from build123d import *

# Parameters (mm, degrees)
BOSS_EXTRUDE1_DEPTH     = 70.5
CUT_EXTRUDE1_DEPTH      = 142.707445111
CUT_EXTRUDE1_DEPTH_BACK = 142.707445111
SKETCH2_R               = 2.5
FILLET1_R               = 1


with BuildPart() as part:
    # Sketch1 → Boss-Extrude1 (new, symmetric)
    with BuildSketch(Plane.XY):
        Polygon((-10, 10), (-3, 10), (-3, 8.272610059), (-5.783778863, 8.272610059), (-5.783778863, 6.747994248), (-3, 4.550753814), (3, 4.550753814), (5.783778863, 6.747994248), (5.783778863, 8.272610059), (3, 8.272610059), (3, 10), (10, 10), (10, 3), (8.272610059, 3), (8.272610059, 5.783778863), (6.747994248, 5.783778863), (4.55, 3.000595152), (4.55, -2.999404848), (6.747994248, -5.783778863), (8.272610059, -5.783778863), (8.272610059, -3), (10, -3), (10, -10), (3, -10), (3, -8.272610059), (5.783778863, -8.272610059), (5.783778863, -6.747994248), (2.999404848, -4.55), (-3.000595152, -4.55), (-5.783778863, -6.747994248), (-5.783778863, -8.272610059), (-3, -8.272610059), (-3, -10), (-10, -10), (-10, -3), (-8.272610059, -3), (-8.272610059, -5.783778863), (-6.747994248, -5.783778863), (-4.55, -3.000595152), (-4.55, 2.999404848), (-6.747994248, 5.783778863), (-8.272610059, 5.783778863), (-8.272610059, 3), (-10, 3), align=None)
    extrude(amount=BOSS_EXTRUDE1_DEPTH, both=True)

    # Sketch2 → Cut-Extrude1 (cut, two sides: drawn at the far end of the back side and taken through both)
    with BuildSketch(Plane.XY.offset(70.5).offset(-CUT_EXTRUDE1_DEPTH_BACK)):
        Circle(SKETCH2_R)
    extrude(amount=CUT_EXTRUDE1_DEPTH + CUT_EXTRUDE1_DEPTH_BACK, mode=Mode.SUBTRACT)

    # Fillet1
    fillet1_edges = [part.edges().sort_by_distance(p)[0] for p in [
        (-10, 10, 0),
        (10, 10, 0),
        (10, -10, 0),
        (-10, -10, 0),
    ]]
    fillet(fillet1_edges, radius=FILLET1_R)


solid = part.part
CAD build for the part. Positions are in the model's coordinates, mm. A direction names the side the tool comes from. Round coordinates to 2 decimals unless told otherwise and drop trailing zeros. Loops run counter-clockwise (first coordinate to the right, second up) from the corner with the lowest first, then second, coordinate; pieces in that order, holes last. Notation, with made-up numbers: M 59.5,18 L 108.5,18 A24 ccw 108.5,28 Z; hole C -32,30 d7. An arc over 180 degrees is marked long. One line per question, with ' | ' between items. Start each with the question number.
Item 1: Pin check, flat tips, straight feed: pin 1 Ø1 at (x, y) = (1.5, 6.5) entering from +Z; pin 2 Ø1.8 at (y, z) = (0.5, 7) entering from +X; pin 3 Ø1.8 at (y, z) = (-1, -33.5) entering from -X. Stop position of each tip, or through.
Item 2: Cut at A-A, the plane y = 0. Write the cut outline in (x, z).
Item 3: Wall check: line 1 (Y direction, x = 8.5, z = -51.5); line 2 (X direction, y = 0, z = 16.5); line 3 (X direction, y = 8, z = -14). Give the ranges that are in metal, low to high.
Item 4: Which spindle directions (+Z, -Z, +X, -X, +Y, -Y) get a long thin tool onto all of the face, cutting with end or side? Do faces 1 (the flat face through (-2, -2, 70.5)), 2 (the flat face through (-10, 6, 1)), 3 (the flat face through (-4.55, 0, 1)), 4 (the flat face through (-4.411, 5.665, 0.987)), 5 (the flat face through (4.55, 0, 1)). Say none if no direction does.
Responses:
1) pin 1: passes through | pin 2: stops at x = 4.55 | pin 3: stops at x = -4.55
2) outline: M -4.55,-70.5 L -2.5,-70.5 L -2.5,70.5 L -4.55,70.5 Z; M 2.5,-70.5 L 4.55,-70.5 L 4.55,70.5 L 2.5,70.5 Z
3) line 1: y = -10 to -3, 3 to 10 | line 2: x = -4.55 to -2.5, 2.5 to 4.55 | line 3: x = -10 to -5.78, 5.78 to 10
4) face 1: +Z, +X, -X, +Y, -Y | face 2: +Z, -Z, -X, +Y, -Y | face 3: +Z, -Z, -X | face 4: +Z, -Z | face 5: +Z, -Z, +X
